Geometry check sheet. Reference: drawing and pictorial views, mm from the part's lowest x, y, z. A direction names the side the tool comes from. Give positions to 0.01 mm unless a question says otherwise; leave off trailing zeros. Write each loop counter-clockwise with the first axis right and the second up, starting at its lowest first coordinate (ties: lowest second). Pieces come first, ordered by that corner, then holes. Notation, with made-up numbers: M 76,40.25 L 84,40.25 A18 ccw 84,57.25 Z; hole C 53,12 d11. An arc over 180 degrees is marked long. Write item = value, one per line. Start each with the question number.
1) Cross-section at B-B, the plane z = 25. Record the cut outline in (x, y).
2) Access from +Z, -Z, +X, -X, +Y, -Y to the whole of each face (thin tool, end or side, straight path). Record for the marked faces 5 and 6.
3) Go/stop test with flat-tipped pins: pin 1 (4.5 mm diameter, centred on x = 37.5, y = 3, fed in from +Z); pin 2 (3 mm diameter, centred on x = 41, y = 4, fed in from -Z); pin 3 (12 mm diameter, centred on x = 21, z = 24.5, fed in from +Y); pin 4 (2 mm diameter, centred on y = 5, z = 28.5, fed in from -X). Record where each tip stops, or that it passes through.
4) Mould release check, pull along X, two halves, no side actions. Record for the marked faces 1, 2, 3 and 4: released by +X, released by -X, zero draft, split by the parting line, or undercut.
5) Scan lines: line 1 along Y through (x, z) = (19.5, 21); line 2 along Z through (x, y) = (15, 7.25); line 3 along Y through (x, z) = (5.5, 70). Record each from-to range of solid material in increasing order. Write a range as [from, to].
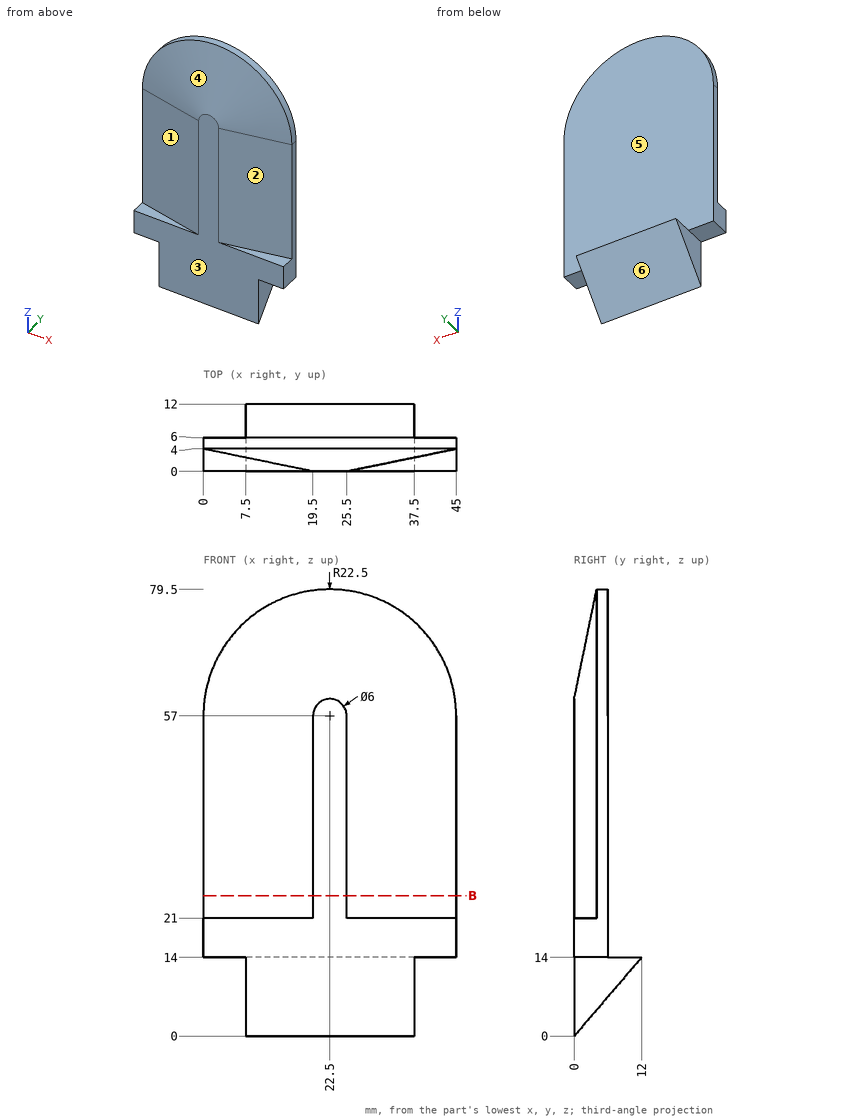
Reply:
q1.outline = M 0,4 L 19.5,0 L 25.5,0 L 45,4 L 45,6 L 0,6 Z
q2.face_5 = +Z, +X, -X, +Y
q2.face_6 = -Z, +X, -X, +Y
q3.pin_1 = 75.38
q3.pin_2 = 14
q3.pin_3 = 6
q3.pin_4 = 0
q4.face_1 = released by -X
q4.face_2 = released by +X
q4.face_3 = zero draft
q4.face_4 = split by the parting line
q5.line_1 = [0, 6]
q5.line_2 = [8.46, 14]
q5.line_3 = [3.77, 6]
